For this review, use the dimensioned drawing (mm, ordinates from the lowest corner) and the shaded views. A direction names the side the tool comes from. Round coordinates to 2 decimals unless told otherwise and drop trailing zeros. Loops run counter-clockwise (first coordinate to the right, second up) from the corner with the lowest first, then second, coordinate; pieces in that order, holes last. Notation, with made-up numbers: (-22.75, 43) -> (-13.75, 43) arc R15 cw to (-13.75, 65) -> close; hole circle Ø11 at (-21, 19). An arc over 180 degrees is marked (long way). Answer as CSV lines item,"result". Start each with the question number.
(1) For P1, Ø1.5, axis at x = 6.5, z = 4, coming from the -Y side; P2, Ø1.5, axis at y = 25.5, z = 5.5, coming from the +X side, all flat-tipped, find the tip position at first contact; note any pin that passes through.
(2) Take a section at C-C, the plane z = 5.25. Write out the cut boundary in (x, y).
(3) Take a section at B-B, the plane y = 8. Write out the cut boundary in (x, z), and give its area (3 significant figures).
(4) Take a section at A-A, the plane x = 11. Write out the cut boundary in (y, z).
(5) Take a section at D-D, the plane x = 19. Write out the cut boundary in (y, z).
(6) To check wall thickness, follow line 1 (X direction, y = 61.1, z = 10); line 2 (Z direction, x = 11, y = 61.9); line 3 (Y direction, x = 0.95, z = 10). State the ranges of each line that lie inside material, in increasing order. Write a range as from..to.
(7) Machinability: for the marked faces 1 and 2, which of the approach directions +Z, -Z, +X, -X, +Y, -Y give a long, thin tool a straight path to every point of the face, cutting with its end or side? Answer none if there is none.
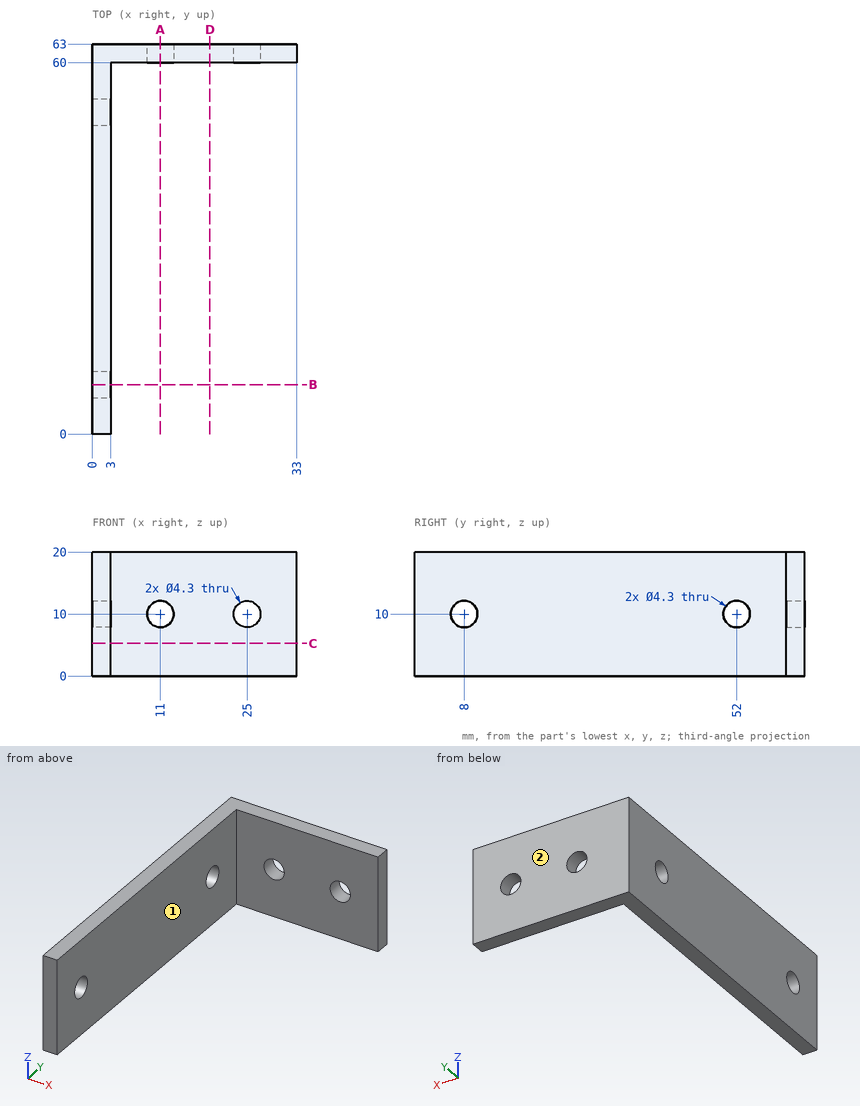
The answers:
1,P1,"y = 60"
1,P2,"x = 3"
2,outline,"(0, 0) -> (3, 0) -> (3, 60) -> (33, 60) -> (33, 63) -> (0, 63) -> close"
3,outline,"(0, 0) -> (3, 0) -> (3, 7.85) -> (0, 7.85) -> close; (0, 12.15) -> (3, 12.15) -> (3, 20) -> (0, 20) -> close"
3,area,"47.1 mm²"
4,outline,"(60, 0) -> (63, 0) -> (63, 7.85) -> (60, 7.85) -> close; (60, 12.15) -> (63, 12.15) -> (63, 20) -> (60, 20) -> close"
5,outline,"(60, 0) -> (63, 0) -> (63, 20) -> (60, 20) -> close"
6,line 1,"0..8.85, 13.15..22.85, 27.15..33"
6,line 2,"0..7.85, 12.15..20"
6,line 3,"0..5.85, 10.15..49.85, 54.15..63"
7,face 1,"+Z, -Z, +X, -Y"
7,face 2,"+Z, -Z, +X, -X, +Y"
